from build123d import *

# Parameters (mm, degrees)
POCKET_DEPTH = 1.002493


with BuildPart() as part:
    # Sketch → Revolution (revolve)
    with BuildSketch(Plane.XZ):
        with BuildLine():
            Line((0, -6), (-1.4, -6))
            Line((-1.4, -6), (-1.4, 0))
            Line((-1.4, 0), (-2.9, 0))
            Line((-2.9, 0), (-2.9, 1.5))
            add(Edge.make_bspline(
                [(0, 2), (-1.27, 2.028858), (-2.9, 1.5)],
                knots=[0, 0, 0, 1, 1, 1], degree=2))
            Line((0, 2), (0, -6))
        make_face()
    revolve(axis=Axis((0, 0, 0), (0, 0, 1)))

    # Sketch001 → Pocket (cut, through all)
    with BuildSketch(Plane.XY.offset(1)):
        Polygon((0.375, 1.5), (-0.375, 1.5), (-0.375, 0.375), (-1.5, 0.375), (-1.5, -0.375), (-0.375, -0.375), (-0.375, -1.5), (0.375, -1.5), (0.375, -0.375), (1.5, -0.375), (1.5, 0.375), (0.375, 0.375), align=None)
    extrude(amount=POCKET_DEPTH, mode=Mode.SUBTRACT)


solid = part.part
Check sheet for the modelled part. Datum: model origin and axes. Units: mm. A direction names the side the tool comes from. Give positions to 0.01 mm unless a question says otherwise; leave off trailing zeros. Write each loop counter-clockwise with the first axis right and the second up, starting at its lowest first coordinate (ties: lowest second). Pieces come first, ordered by that corner, then holes. Notation, with made-up numbers: (49.5, 50.25) -> (66.5, 50.25) arc R15 cw to (66.5, 55.25) -> close; hole circle Ø9 at (62.5, 67.5). An arc over 180 degrees is marked (long way). Use one line per item in the form item = value. Start each with the question number.
1. Access from +Z, -Z, +X, -X, +Y, -Y to the whole of each face (thin tool, end or side, straight path). Record for faces 1 (the flat face through (-0.375, 0.9, 1.5)), 2 (the cylindrical face through (2.9, -0.1, 0.8)).
2. Mould release check, pull along X, two halves, no side actions. Record for faces 3 (the flat face through (-0.9, 0.375, 1.5)), 4 (the flat face through (0, 0, -6)), 5 (the cylindrical face through (1.4, -0.06, -2.96)): pulls with the +X half, pulls with the -X half, needs draft (parallel to the pull), parting line crosses it, or undercut.
3. Go/stop test with flat-tipped pins: P1, Ø0.5, axis at y = -1, z = 1.5, coming from the -X side; P2, Ø3, axis at x = -2.5, y = 1.5, coming from the +Z side; P3, Ø1.1, axis at x = 1, z = 1.5, coming from the +Y side; P4, Ø0.9, axis at x = -0.5, y = 0, coming from the +Z side. Record where each tip stops, or that it passes through.
4. Section check A-A (z = -1.5). Record the cut outline in (x, y), and give its area (3 significant figures).
5. Thickness scan on line 1 along Z through (x, y) = (0.2, 1.2); line 2 along Y through (x, z) = (-0.05, -1.5); line 3 along Y through (x, z) = (-1.65, 1.25). Record the ranges inside material, lowest first. Write a range as from..to.
Conclusion:
q1.face_1 = +Z
q1.face_2 = +Z, -Z
q2.face_3 = undercut
q2.face_4 = needs draft
q2.face_5 = parting line crosses it
q3.P1 = -2.8
q3.P2 = 1.88
q3.P3 = 2.86
q3.P4 = 1.99
q4.outline = circle Ø2.8 at (0, 0)
q4.area = 6.16 mm²
q5.line_1 = -6..1
q5.line_2 = -1.4..1.4
q5.line_3 = -2.38..2.38
